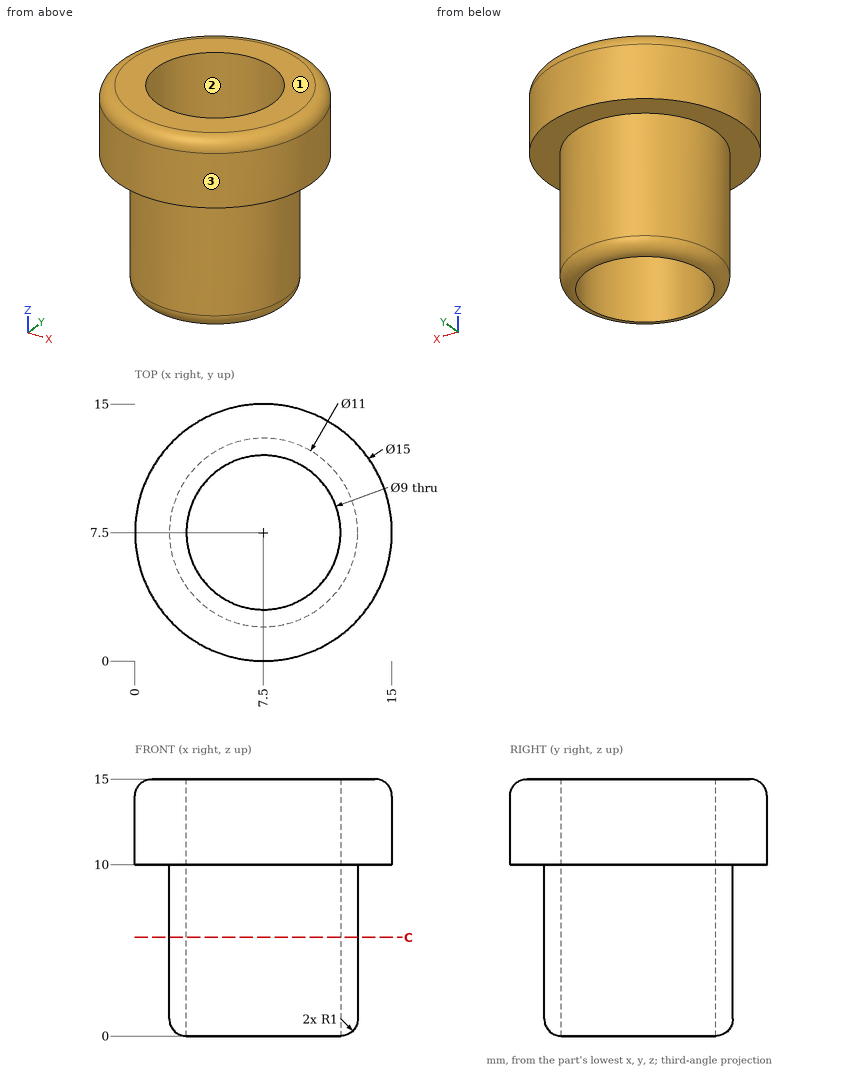
Here's the drawing with two shaded views (mm, measured from the low corner). I have some questions. Give positions to 0.01 mm unless a question says otherwise; leave off trailing zeros. Loops run counter-clockwise (first coordinate to the right, second up) from the corner with the lowest first, then second, coordinate; pieces in that order, holes last. Notation, with made-up numbers: M -8.5,49.25 L 33.5,49.25 A32 cw 33.5,83.25 Z; hole C -31.75,72 d4. An arc over 180 degrees is marked long. Answer in a Markdown table with one row per item.
1. If I drill on line 1 along Y through (x, z) = (7.5, 11.5); line 2 along Y through (x, z) = (7.5, 8.5); line 3 along Z through (x, y) = (10, 2.25), over which ranges is the centre line in solid material (lowest first)?
Taken from the geometry:
| item | result |
|---|---|
| line 1 | y = 0 to 3, 12 to 15 |
| line 2 | y = 2 to 3, 12 to 13 |
| line 3 | z = 10 to 15 |
2. For pin 1 Ø2 at (x, z) = (7, 8) entering from -Y; pin 2 Ø8 at (x, y) = (12, 8.5) entering from -Z; pin 3 Ø1.5 at (y, z) = (8.5, 12) entering from -X, each with a flat end and sliding along its axis, tell me the tip position at first contact or that it passes through.
Taken from the geometry:
| item | result |
|---|---|
| pin 1 | stops at y = 2 |
| pin 2 | stops at z = 0 |
| pin 3 | stops at x = 0 |
3. Suppose I cut it at C-C on z = 5.75. Write out the boundary of the cut face in (x, y).
Taken from the geometry:
| item | result |
|---|---|
| outline | C 7.5,7.5 d11; hole C 7.5,7.5 d9 |
4. Thinking about a two-plate mould opening in X: for the marked faces 1, 2 and 3, which applies, released by +X, released by -X, zero draft, split by the parting line, or undercut?
Taken from the geometry:
| item | result |
|---|---|
| face 1 | zero draft |
| face 2 | undercut |
| face 3 | split by the parting line |
